Work out the finished part from the listing and answer in its coordinate system (mm). Face numbers are marked on the shaded views. A direction names the side the tool comes from. Coordinates: 2 decimals unless noted, no trailing zeros. Loops run counter-clockwise (first coordinate to the right, second up) from the corner with the lowest first, then second, coordinate; pieces in that order, holes last. Notation, with made-up numbers: (21.5, 87.25) -> (57.5, 87.25) arc R12 ccw to (57.5, 106.25) -> close; hole circle Ø6 at (80, 43.25). An arc over 180 degrees is marked (long way). One line per question, with ' | ' between items.
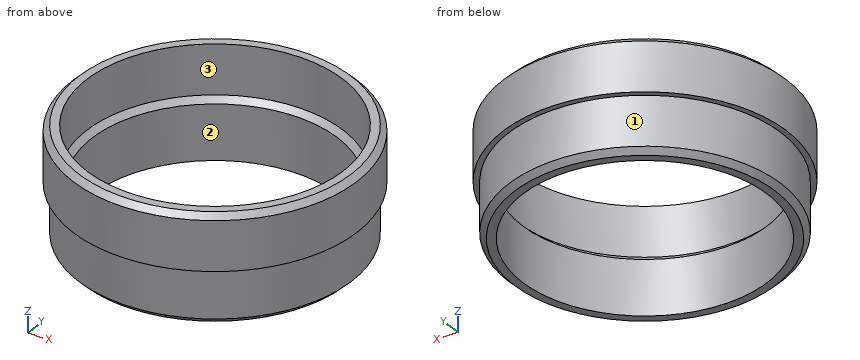
Autodesk Inventor part; units mm, degrees
ref_plane "YZ Plane" through (0, 0, 0) normal (1, 0, 0) x (0, 1, 0)
ref_plane "XZ Plane" through (0, 0, 0) normal (0, 1, 0) x (-1, 0, 0)
ref_plane "XY Plane" through (0, 0, 0) normal (0, 0, 1) x (1, 0, 0)
sketch "Sketch1" plane through (0, 0, 0) normal (0, 0, 1) x (1, 0, 0)
  circle A0 centre (0, 0) radius 12.4625
  circle A1 centre (0, 0) radius 12.9625
  circle A2 centre (0, 0) radius 11.7125
  circle A3 centre (0, 0) radius 11.2125
  dimension "d0" = 24.925
  dimension "d1" = 25.925
  dimension "d2" = 1.25
  dimension "d3" = 1.25
extrude "Extrusion1" add sketch "Sketch1" along normal blind 5 contours A0 | A1
extrude "Extrusion2" add sketch "Sketch1" against normal blind 5 contours A0 | A2
chamfer "Chamfer1" distance 0.5 angle 45 1 edges at (-11.7125, 0, 0)
chamfer "Chamfer2" distance 0.5 angle 45 2 edges at (-12.4625, 0, -5) (-12.9625, 0, 5)
properties part number "Camera Mount Adapter"
1) Find section D-D (z = 2.5). Write down the section's boundary in (x, y) (1 decimal).
Check values:
outline: circle Ø25.9 at (0, 0); hole circle Ø23.4 at (0, 0)
2) Find the intervals of material crossed by line 1 along Y through (x, z) = (0, 2.65); line 2 along Y through (x, z) = (0, -4); line 3 along X through (y, z) = (-3.5, -3.75), in increasing order.
Check values:
line 1: y = -12.96 to -11.71, 11.71 to 12.96 | line 2: y = -12.46 to -11.21, 11.21 to 12.46 | line 3: x = -11.96 to -10.65, 10.65 to 11.96
3) Find section C-C (z = -4). Write down the section's boundary in (x, y) (1 decimal).
Check values:
outline: circle Ø24.9 at (0, 0); hole circle Ø22.4 at (0, 0)
4) For the marked faces 1, 2 and 3, determine the directions among +Z, -Z, +X, -X, +Y, -Y from which every point of the face is accessible in a straight line to the end or side of a thin tool.
Check values:
face 1: -Z | face 2: +Z, -Z | face 3: +Z
5) Flat-ended cylindrical pins translate along their axes: pin 1 (2 mm diameter, centred on x = 7.5, z = 3, fed in from -Y) (3 decimals); pin 2 (4 mm diameter, centred on x = 4.5, y = -8.5, fed in from +Z); pin 3 (5 mm diameter, centred on x = -9, z = 1.5, fed in from +Y) (3 decimals). Find the tip coordinate at first contact, or state that the pin passes through.
Check values:
pin 1: stops at y = -11.215 | pin 2: stops at z = 0.4 | pin 3: stops at y = 11.215
